```python
from build123d import *

# Parameters (mm, degrees)
F0_W      = 127
F0_H      = 101.6
F1_DEPTH  = 9.525
F1_FACE_W = 127
F1_FACE_H = 101.6
F2_DEPTH  = 9.525
F3_W      = 50.8
F3_H      = 50.8
F3_R      = 9.525
F4_DEPTH  = 25.4
F5_R      = 5.08
F6_R      = 6.35
F7_DEPTH  = 116.078


with BuildPart() as f1:
    # F0 (on Top) → F1 (new body)
    with BuildSketch(Plane.XY):
        Rectangle(F0_W, F0_H)
    extrude(amount=F1_DEPTH)

    # F1_face (on face) → F2 (join)
    with BuildSketch(Plane(origin=(0, 0, 0), x_dir=(1, 0, 0), z_dir=(0, 0, -1))):
        Rectangle(F1_FACE_W, F1_FACE_H)
    extrude(amount=F2_DEPTH)

    # F3 (on face) → F4 (cut)
    with BuildSketch(Plane.XY.offset(9.525)):
        Rectangle(F3_W, F3_H)
        with Locations((-44.45, -31.75)):
            Circle(F3_R)
        with Locations((-44.45, 31.75)):
            Circle(F3_R)
        with Locations((44.45, 31.75)):
            Circle(F3_R)
        with Locations((44.45, -31.75)):
            Circle(F3_R)
    extrude(amount=-F4_DEPTH, mode=Mode.SUBTRACT)

    # F5
    f5_edges = [f1.edges().sort_by_distance(p)[0] for p in [
        (-25.4, 25.4, 0),
        (-25.4, -25.4, 0),
        (25.4, -25.4, 0),
        (25.4, 25.4, 0),
    ]]
    fillet(f5_edges, radius=F5_R)

    # F6 (on face) → F7 (cut)
    with BuildSketch(Plane.XZ.offset(50.8)):
        Circle(F6_R)
    extrude(amount=-F7_DEPTH, mode=Mode.SUBTRACT)


solid = f1.part
```
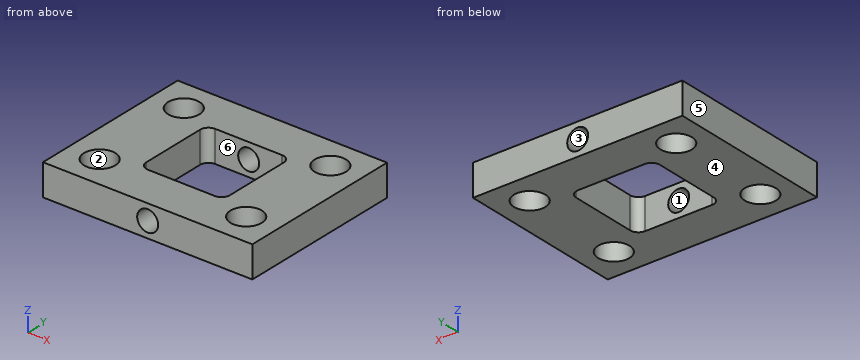
Design review of the part built by this model. Coordinates are the model's own, in mm. Face numbers are marked on the shaded views. A direction names the side the tool comes from. Round coordinates to 2 decimals unless told otherwise and drop trailing zeros. Write each loop counter-clockwise with the first axis right and the second up, starting at its lowest first coordinate (ties: lowest second). Pieces come first, ordered by that corner, then holes. Notation, with made-up numbers: (64, 8) -> (78, 8) arc R32 cw to (78, 46) -> close; hole circle Ø9 at (9, 1). An arc over 180 degrees is marked (long way). Answer in a Markdown table with one row per item.
Q1. Take a section at A-A, the plane y = -31.75. State the section outline as (x, z) points (3 decimals), then the cut area to 3 significant figures.
The answers:
| item | result |
|---|---|
| outline | (-63.5, -9.525) -> (-53.975, -9.525) -> (-53.975, 9.525) -> (-63.5, 9.525) -> close; (-34.925, -9.525) -> (34.925, -9.525) -> (34.925, 9.525) -> (-34.925, 9.525) -> close; (53.975, -9.525) -> (63.5, -9.525) -> (63.5, 9.525) -> (53.975, 9.525) -> close; hole circle Ø12.7 at (0, 0) |
| area | 1,570 mm² |
Q2. Clearance check with flat-ended pins moving along their axes: pin 1 Ø17 at (x, y) = (44.45, -31.75) entering from -Z; pin 2 Ø25 at (x, y) = (-44.45, 31.75) entering from -Z (3 decimals). State where each tip first meets the part, or that it passes through.
The answers:
| item | result |
|---|---|
| pin 1 | through |
| pin 2 | z = -9.525 |
Q3. For the marked faces 5 and 6, list the 3-axis set-ups (+Z, -Z, +X, -X, +Y, -Y) from which the entire face can be reached by the end or side of a thin tool; tool diameter is ignored.
The answers:
| item | result |
|---|---|
| face 5 | +Z, -Z, -X, +Y, -Y |
| face 6 | +Z, -Z |
Q4. Draft analysis for pull direction Z (two halves, no side actions). For the marked faces 1, 2, 3 and 4, state which applies: +Z half, -Z half, draft (parallel to the pull), parting line (faces both ways), or undercut.
The answers:
| item | result |
|---|---|
| face 1 | undercut |
| face 2 | draft |
| face 3 | undercut |
| face 4 | -Z half |
Q5. Take a section at B-B, the plane z = 0. State the section outline as (x, y) points (3 decimals).
The answers:
| item | result |
|---|---|
| outline | (-63.5, -50.8) -> (-6.35, -50.8) -> (-6.35, -25.4) -> (-20.32, -25.4) arc R5.08 cw to (-25.4, -20.32) -> (-25.4, 20.32) arc R5.08 cw to (-20.32, 25.4) -> (-6.35, 25.4) -> (-6.35, 50.8) -> (-63.5, 50.8) -> close; (6.35, -50.8) -> (63.5, -50.8) -> (63.5, 50.8) -> (6.35, 50.8) -> (6.35, 25.4) -> (20.32, 25.4) arc R5.08 cw to (25.4, 20.32) -> (25.4, -20.32) arc R5.08 cw to (20.32, -25.4) -> (6.35, -25.4) -> close; hole circle Ø19.05 at (-44.45, -31.75); hole circle Ø19.05 at (-44.45, 31.75); hole circle Ø19.05 at (44.45, -31.75); hole circle Ø19.05 at (44.45, 31.75) |
Q6. Take a section at D-D, the plane y = 12.5. State the section outline as (x, z) points (3 decimals).
The answers:
| item | result |
|---|---|
| outline | (-63.5, -9.525) -> (-25.4, -9.525) -> (-25.4, 9.525) -> (-63.5, 9.525) -> close; (25.4, -9.525) -> (63.5, -9.525) -> (63.5, 9.525) -> (25.4, 9.525) -> close |
Q7. Take a section at C-C, the plane x = 0. State the section outline as (y, z) points (3 decimals), then the cut area to 3 significant figures.
The answers:
| item | result |
|---|---|
| outline | (-50.8, -9.525) -> (-25.4, -9.525) -> (-25.4, -6.35) -> (-50.8, -6.35) -> close; (-50.8, 6.35) -> (-25.4, 6.35) -> (-25.4, 9.525) -> (-50.8, 9.525) -> close; (25.4, -9.525) -> (50.8, -9.525) -> (50.8, -6.35) -> (25.4, -6.35) -> close; (25.4, 6.35) -> (50.8, 6.35) -> (50.8, 9.525) -> (25.4, 9.525) -> close |
| area | 323 mm² |
Q8. To check wall thickness, follow L1, parallel to Y at x = 44.45, z = -1.75 (3 decimals); L2, parallel to Y at x = 20, z = -5.75; L3, parallel to X at y = 3, z = 3.25. State the ranges of each line that lie inside material, in increasing order. Write a range as [from, to].
The answers:
| item | result |
|---|---|
| L1 | [-50.8, -41.275], [-22.225, 22.225], [41.275, 50.8] |
| L2 | [-50.8, -25.4], [25.4, 50.8] |
| L3 | [-63.5, -25.4], [25.4, 63.5] |
